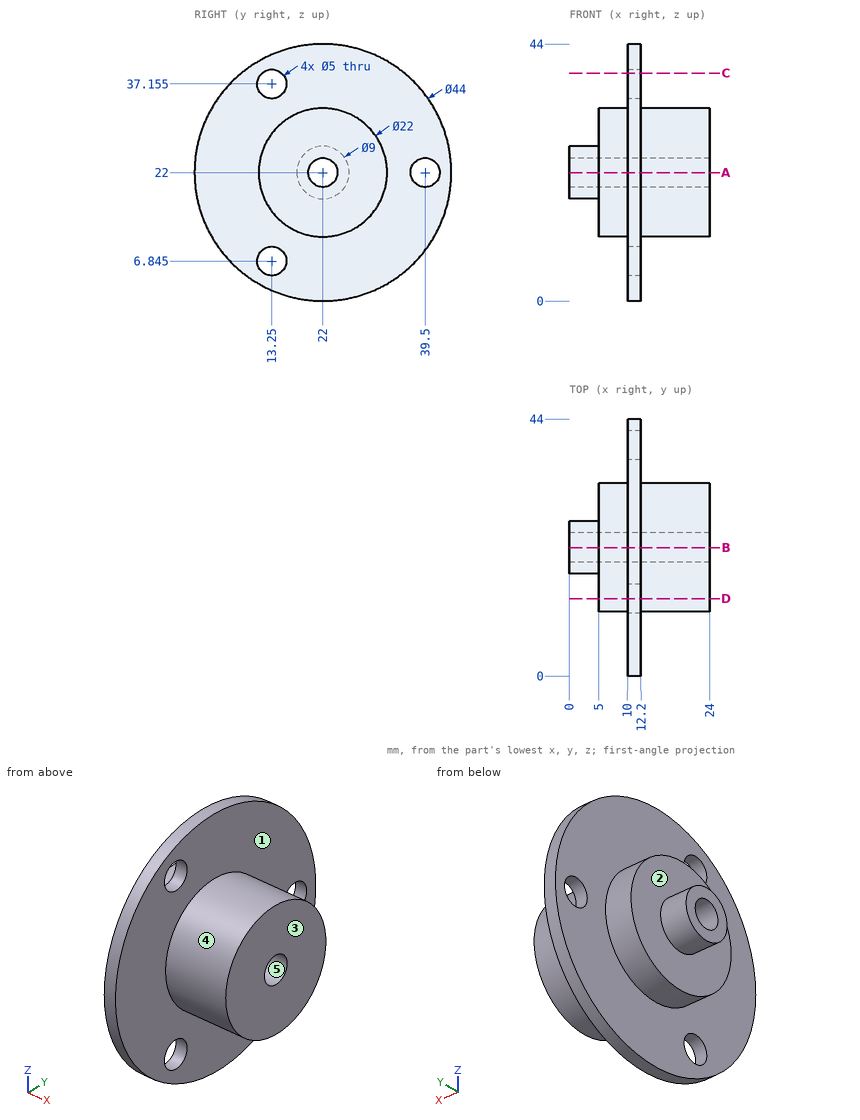
Part print with two shaded views. Sizes in mm from the minimum x, y, z corner. A direction names the side the tool comes from. Round coordinates to 2 decimals unless told otherwise and drop trailing zeros. Write each loop counter-clockwise with the first axis right and the second up, starting at its lowest first coordinate (ties: lowest second). Pieces come first, ordered by that corner, then holes. Notation, with made-up numbers: (-5, -5.5) - (49, -5.5) arc R23 ccw to (49, 3.5) - close; hole circle Ø2 at (60, 9.5). An arc over 180 degrees is marked (long way). Use CSV: the item, a comma, the result in double quotes.
Item 1: Flat gauge pins, fed straight in: P1, Ø3, axis at x = 13.5, y = 33, coming from the +Z side (1 decimal); P2, Ø12, axis at x = 19.5, z = 24.5, coming from the +Y side; P3, Ø1.5, axis at y = 32, z = 38.5, coming from the -X side. Where does each tip first touch, or does it go through?
Results list:
P1,"stops at z = 41.5"
P2,"stops at y = 33"
P3,"stops at x = 10"
Item 2: Slice it at B-B, the plane y = 22. Write the cut outline in (x, z).
Results list:
outline,"(0, 17.5) - (5, 17.5) - (5, 11) - (10, 11) - (10, 0) - (12.2, 0) - (12.2, 11) - (24, 11) - (24, 19.5) - (0, 19.5) - close; (0, 24.5) - (24, 24.5) - (24, 33) - (12.2, 33) - (12.2, 44) - (10, 44) - (10, 33) - (5, 33) - (5, 26.5) - (0, 26.5) - close"
Item 3: Slice it at C-C, the plane z = 39. Write the cut outline in (x, y) (1 decimal).
Results list:
outline,"(10, 8) - (12.2, 8) - (12.2, 11.6) - (10, 11.6) - close; (10, 14.9) - (12.2, 14.9) - (12.2, 36) - (10, 36) - close"
Item 4: Slice it at D-D, the plane y = 13.25. Write the cut outline in (x, z) (1 decimal).
Results list:
outline,"(5, 15.3) - (10, 15.3) - (10, 9.3) - (12.2, 9.3) - (12.2, 15.3) - (24, 15.3) - (24, 28.7) - (12.2, 28.7) - (12.2, 34.7) - (10, 34.7) - (10, 28.7) - (5, 28.7) - close; (10, 1.8) - (12.2, 1.8) - (12.2, 4.3) - (10, 4.3) - close; (10, 39.7) - (12.2, 39.7) - (12.2, 42.2) - (10, 42.2) - close"
Item 5: Tool access for the marked faces 1 and 2: list every direction of +Z, -Z, +X, -X, +Y, -Y with a clear straight run to the whole face (end or side of a thin tool).
Results list:
face 1,"+X"
face 2,"-X"
Item 6: Slice it at A-A, the plane z = 22. Write the cut outline in (x, y).
Results list:
outline,"(0, 17.5) - (5, 17.5) - (5, 11) - (10, 11) - (10, 0) - (12.2, 0) - (12.2, 11) - (24, 11) - (24, 19.5) - (0, 19.5) - close; (0, 24.5) - (24, 24.5) - (24, 33) - (12.2, 33) - (12.2, 37) - (10, 37) - (10, 33) - (5, 33) - (5, 26.5) - (0, 26.5) - close; (10, 42) - (12.2, 42) - (12.2, 44) - (10, 44) - close"
Item 7: Wall check: L1, parallel to Y at x = 10.55, z = 22; L2, parallel to X at y = 37.5, z = 12.5; L3, parallel to X at y = 12, z = 19.5. Give the ranges that are in metal, low to high.
Results list:
L1,"y = 0 to 19.5, 24.5 to 37, 42 to 44"
L2,"x = 10 to 12.2"
L3,"x = 5 to 24"
Item 8: Pull direction Y, two halves, no side cores. Call the marked faces 3, 4 and 5: pulls with the +Y half, pulls with the -Y half, needs draft (parallel to the pull), parting line crosses it, or undercut.
Results list:
face 3,"needs draft"
face 4,"parting line crosses it"
face 5,"undercut"
